Check sheet for the drawn part. Datum: minimum x, y, z corner. Units: mm. A direction names the side the tool comes from. Coordinates: 2 decimals unless noted, no trailing zeros. Loops run counter-clockwise (first coordinate to the right, second up) from the corner with the lowest first, then second, coordinate; pieces in that order, holes last. Notation, with made-up numbers: (-40, 81) - (-8, 81) arc R15 cw to (-8, 103) - close; hole circle Ø7 at (63.25, 29). An arc over 180 degrees is marked (long way). Answer as CSV lines item,"result". Start each with the question number.
1. Set-up check for the marked faces 1, 2, 3 and 4: record each of +Z, -Z, +X, -X, +Y, -Y from which the full face is reachable in a straight line by a thin tool's end or side.
2. Gauge pin test, flat ends, axial feed: P1, Ø4, axis at y = 5, z = 15.5, coming from the -X side; P2, Ø1.5, axis at y = 5.5, z = 8.5, coming from the +X side; P3, Ø0.6, axis at x = 1.5, z = 10.5, coming from the -Y side. Record the tip position at first contact, or that the pin passes through.
3. Cross-section at C-C (x = 12.5). Enter the section's corners in (y, z).
4. Material ranges on line 1 (Z direction, x = 50, y = 0.9); line 2 (X direction, y = 0.9, z = 2); line 3 (X direction, y = 2.75, z = 20.25), recorded low to high. Write a range as [from, to].
5. Cross-section at B-B (y = 0.75). Enter the section's corners in (x, z).
6. Cross-section at D-D (z = 6.75). Enter the section's corners in (x, y).
7. Cross-section at A-A (z = 2). Enter the section's corners in (x, y), plus the area to 3 significant figures.
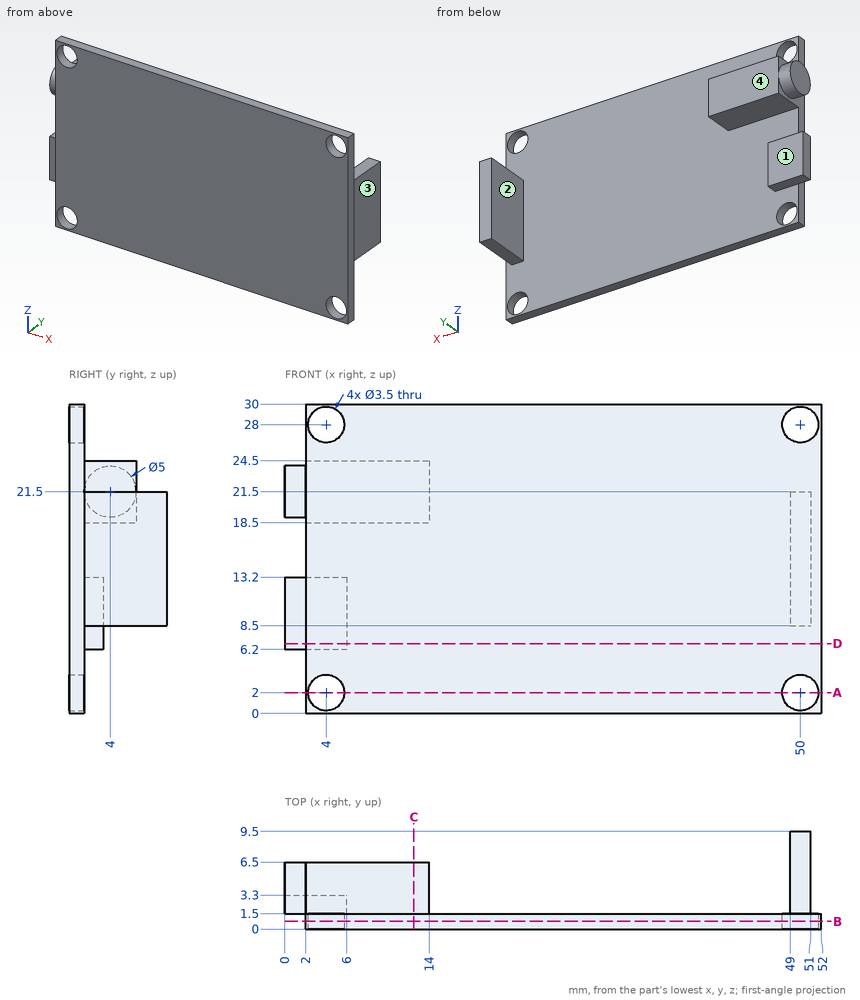
Values follow:
1,face 1,"-Z, -X, +Y"
1,face 2,"+Z, -Z, +Y"
1,face 3,"+Z, -Z, +X, +Y"
1,face 4,"+Z, -Z, -X, +Y"
2,P1,"stops at x = 49"
2,P2,"stops at x = 51"
2,P3,"stops at y = 1.5"
3,outline,"(0, 0) - (1.5, 0) - (1.5, 18.5) - (6.5, 18.5) - (6.5, 24.5) - (1.5, 24.5) - (1.5, 30) - (0, 30) - close"
4,line 1,"z = [0, 0.25], [3.75, 26.25], [29.75, 30]"
4,line 2,"x = [2, 2.25], [5.75, 48.25], [51.75, 52]"
4,line 3,"x = [0, 14], [49, 51]"
5,outline,"(2, 0) - (52, 0) - (52, 30) - (2, 30) - close; hole circle Ø3.5 at (4, 2); hole circle Ø3.5 at (4, 28); hole circle Ø3.5 at (50, 2); hole circle Ø3.5 at (50, 28)"
6,outline,"(0, 1.5) - (2, 1.5) - (2, 0) - (52, 0) - (52, 1.5) - (6, 1.5) - (6, 3.3) - (0, 3.3) - close"
7,outline,"(2, 0) - (2.25, 0) - (2.25, 1.5) - (2, 1.5) - close; (5.75, 0) - (48.25, 0) - (48.25, 1.5) - (5.75, 1.5) - close; (51.75, 0) - (52, 0) - (52, 1.5) - (51.75, 1.5) - close"
7,area,"64.5 mm²"
